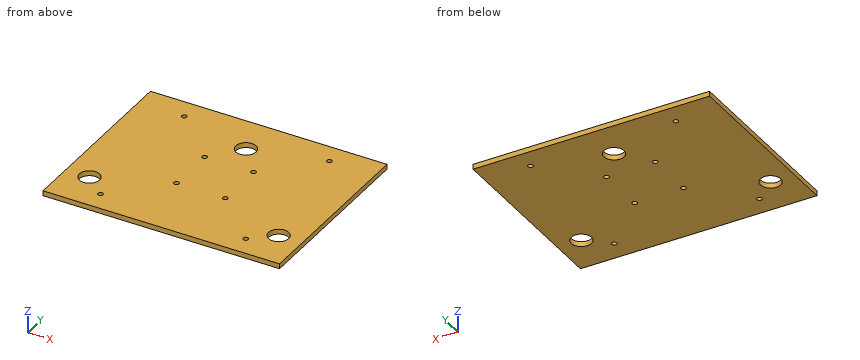
Autodesk Fusion 360 part; units mm, degrees
sketch "movingPlatform" plane through (0, 0, 0) normal (0, 0, 1) x (1, 0, 0)
  line L0 (-75, 59) -> (75, 59)
  line L1 (75, 59) -> (75, -59)
  line L2 (75, -59) -> (-75, -59)
  line L3 (-75, -59) -> (-75, 59)
  line L4 (-75, 59) -> (75, -59) construction
  line L5 (75, 59) -> (-75, -59) construction
  circle A0 centre (-60, -34) radius 6.4
  line L6 (0, 2.5) -> (0, 20)
  circle A1 centre (60, -34) radius 6.4
  circle A2 centre (0, 34) radius 6.4
  circle A3 centre (-46, -46) radius 1.588
  circle A4 centre (-15.5, -15.5) radius 1.588
  circle A5 centre (0, 0) radius 57 construction
  circle A6 centre (15.5, -15.5) radius 1.588
  circle A7 centre (15.5, 15.5) radius 1.588
  circle A8 centre (46, -46) radius 1.588
  circle A9 centre (-46, 46) radius 1.588
  circle A10 centre (46, 46) radius 1.588
  circle A11 centre (-15.5, 15.5) radius 1.588
  dimension "d1" = 150
  dimension "d2" = 118
  dimension "d3" = 12.8
  dimension "d4" = 120
  dimension "d5" = 12.8
  dimension "d6" = 68
  dimension "d7" = 25
  dimension "d8" = 25
  dimension "d9" = 3.176
  dimension "d12" = 92
  dimension "d13" = 92
  dimension "d21" = 3.176
  dimension "d24" = 31
  dimension "d25" = 31
  dimension "d27" = 15.5
  dimension "d31" = 114
  dimension "d34" = 46
  dimension "d37" = 46
  dimension "d49" = 15.5
extrude "Extrude3" add sketch "movingPlatform" along normal blind 3.175
equation "d4 = 132.800 mm - 12.8 mm"
Here's how the part is built. I have some questions about the finished solid (model axes, mm). Round coordinates to 2 decimals unless told otherwise and drop trailing zeros. Order: outer loops, then holes, each group sorted by start corner. A loop starts at its lowest first (then second) coordinate and runs counter-clockwise, first axis right, second up. Notation, with made-up numbers: M 19,14.5 L 35,14.5 A7 cw 35,23.5 Z; hole C 11.25,52 d11. An arc over 180 degrees is marked long. One line per question, with ' | ' between items.
1) Imagine slicing it at D-D, the plane x = -15.5. Write out the boundary of the cut face in (y, z) (3 decimals).
Checked values:
outline: M -59,0 L -17.088,0 L -17.088,3.175 L -59,3.175 Z; M -13.912,0 L 13.912,0 L 13.912,3.175 L -13.912,3.175 Z; M 17.088,0 L 59,0 L 59,3.175 L 17.088,3.175 Z
2) Imagine slicing it at A-A, the plane y = -15.5. Write out the boundary of the cut face in (x, z) (3 decimals).
Checked values:
outline: M -75,0 L -17.088,0 L -17.088,3.175 L -75,3.175 Z; M -13.912,0 L 13.912,0 L 13.912,3.175 L -13.912,3.175 Z; M 17.088,0 L 75,0 L 75,3.175 L 17.088,3.175 Z
3) Imagine slicing it at B-B, the plane x = 60. Write out the boundary of the cut face in (y, z) (3 decimals), plus the area to 3 significant figures.
Checked values:
outline: M -59,0 L -40.4,0 L -40.4,3.175 L -59,3.175 Z; M -27.6,0 L 59,0 L 59,3.175 L -27.6,3.175 Z | area: 334 mm²
4) Imagine slicing it at C-C, the plane z = 1.3. Count the separate pieces of the cut face and the enclosed holes in it, plus the area to 3 significant figures.
Checked values:
separate pieces: 1 | enclosed holes: 11 | area: 17,300 mm²
5) I'm going to push a flat-ended pin straight in: pin 1 Ø1.9 at (x, y) = (-46, 46) entering from +Z (3 decimals). Where does the tip first touch, or does it pass through?
Checked values:
pin 1: passes through
6) I need wall thicknesses on line 1 (Y direction, x = -15.5, z = 1.4); line 2 (X direction, y = 34.5, z = 2.45); line 3 (Y direction, x = -60, z = 1.45). Which ranges of each line are inside material? Lowest first, please.
Checked values:
line 1: y = -59 to -17.09, -13.91 to 13.91, 17.09 to 59 | line 2: x = -75 to -6.38, 6.38 to 75 | line 3: y = -59 to -40.4, -27.6 to 59
